Check sheet for the modelled part. Datum: model origin and axes. Units: mm. A direction names the side the tool comes from. Give positions to 0.01 mm unless a question says otherwise; leave off trailing zeros. Loops run counter-clockwise (first coordinate to the right, second up) from the corner with the lowest first, then second, coordinate; pieces in that order, holes last. Notation, with made-up numbers: (2.5, -23) - (35.5, -23) arc R22 ccw to (35.5, -4) - close; hole circle Ø5 at (46, 8.25). An arc over 180 degrees is marked (long way). Use CSV: the item, a comma, the result in double quotes.
from build123d import *

# Parameters (mm, degrees)
ESBO_O1_W                  = 90.2
ESBO_O1_H                  = 95.9
RESSALTO_EXTRUS_O1_DEPTH   = 3.5
ESBO_O2_R                  = 1.25
CORTE_EXTRUS_O1_DEPTH      = 5
CORTE_EXTRUS_O3_DEPTH      = 5
ESBO_O4_R                  = 1.25
CORTE_EXTRUS_O2_DEPTH      = 10
CHANFRO4_SIZE              = 1.75
CHANFRO5_SIZE              = 1.75
CHANFRO6_SIZE              = 2.25
CHANFRO7_SIZE              = 2.25
CORTE_EXTRUS_O4_DEPTH      = 0.2
CORTE_EXTRUS_O5_DEPTH      = 0.2
CORTE_EXTRUS_O7_DEPTH      = 66.920122118
CORTE_EXTRUS_O7_DEPTH_BACK = 5
ESBO_O7_W                  = 1.6
ESBO_O7_H                  = 6.5
ESBO_O8_W                  = 1.6
ESBO_O8_H                  = 6.5
CORTE_EXTRUS_O8_DEPTH      = 5


with BuildPart() as part:
    # Esboço1 → Ressalto-extrusão1 (new body)
    with BuildSketch(Plane.XY):
        Rectangle(ESBO_O1_W, ESBO_O1_H)
    extrude(amount=RESSALTO_EXTRUS_O1_DEPTH)

    # Esboço2 → Corte-extrusão1 (cut)
    with BuildSketch(Plane.XY):
        with Locations((-36.2, 42.85)):
            Circle(ESBO_O2_R)
        with Locations((37.5, 42.85)):
            Circle(ESBO_O2_R)
        with Locations((40, -42.85)):
            Circle(ESBO_O2_R)
        with Locations((-40, -42.85)):
            Circle(ESBO_O2_R)
    extrude(amount=CORTE_EXTRUS_O1_DEPTH, mode=Mode.SUBTRACT)

    # Esboço3 → Corte-extrusão3 (cut)
    with BuildSketch(Plane.XY):
        Polygon((-26.25, 41.25), (26.25, 41.25), (41.25, 26.25), (41.25, -26.25), (26.25, -41.25), (-26.25, -41.25), (-41.25, -26.25), (-41.25, 26.25), align=None)
    extrude(amount=CORTE_EXTRUS_O3_DEPTH, mode=Mode.SUBTRACT)

    # Esboço4 → Corte-extrusão2 (cut)
    with BuildSketch(Plane.XY):
        with Locations((-36.25, 36.25)):
            Circle(ESBO_O4_R)
        with Locations((36.25, 36.25)):
            Circle(ESBO_O4_R)
        with Locations((-36.25, -36.25)):
            Circle(ESBO_O4_R)
        with Locations((36.25, -36.25)):
            Circle(ESBO_O4_R)
    extrude(amount=CORTE_EXTRUS_O2_DEPTH, mode=Mode.SUBTRACT)

    # Chanfro4
    chanfro4_edges = [part.edges().sort_by_distance(p)[0] for p in [
        (-41.25, -42.85, 3.5),
    ]]
    chamfer(chanfro4_edges, length=CHANFRO4_SIZE)

    # Chanfro5
    chanfro5_edges = [part.edges().sort_by_distance(p)[0] for p in [
        (38.75, -42.85, 3.5),
    ]]
    chamfer(chanfro5_edges, length=CHANFRO5_SIZE)

    # Chanfro6
    chanfro6_edges = [part.edges().sort_by_distance(p)[0] for p in [
        (-37.45, 42.85, 3.5),
    ]]
    chamfer(chanfro6_edges, length=CHANFRO6_SIZE)

    # Chanfro7
    chanfro7_edges = [part.edges().sort_by_distance(p)[0] for p in [
        (36.25, 42.85, 3.5),
    ]]
    chamfer(chanfro7_edges, length=CHANFRO7_SIZE)

    # Esboço5 → Corte-extrusão4 (cut)
    with BuildSketch(Plane.XY.offset(3.5)):
        Polygon((-34.011664728, -41.359633286), (-33.364529311, -41.359633286), (-33.364529311, -44.859633286), (-33.678631875, -44.859633286), (-33.678631875, -41.718607645), (-34.217093414, -41.718607645), align=None)
    extrude(amount=-CORTE_EXTRUS_O4_DEPTH, mode=Mode.SUBTRACT)

    # Esboço6 → Corte-extrusão5 (cut)
    with BuildSketch(Plane(origin=(0, 0, 0), x_dir=(-1, 0, 0), z_dir=(0, 0, -1))):
        Polygon((33.93825461, -40.504659527), (34.585390027, -40.504659527), (34.585390027, -44.004659527), (34.271287463, -44.004659527), (34.271287463, -40.863633886), (33.732825924, -40.863633886), align=None)
    extrude(amount=-CORTE_EXTRUS_O5_DEPTH, mode=Mode.SUBTRACT)

    # Esboço7 → Corte-extrusão7 (cut, two sides: drawn at the far end of the back side and taken through both)
    with BuildSketch(Plane(origin=(0, 0, 0), x_dir=(-1, 0, 0), z_dir=(0, 0, -1)).offset(-CORTE_EXTRUS_O7_DEPTH_BACK)):
        with Locations((-44.3, -44.7)):
            Rectangle(ESBO_O7_W, ESBO_O7_H)
    extrude(amount=CORTE_EXTRUS_O7_DEPTH + CORTE_EXTRUS_O7_DEPTH_BACK, mode=Mode.SUBTRACT)

    # Esboço8 → Corte-extrusão8 (cut)
    with BuildSketch(Plane.XY.offset(3.5)):
        with Locations((-44.3, 44.7)):
            Rectangle(ESBO_O8_W, ESBO_O8_H)
    extrude(amount=-CORTE_EXTRUS_O8_DEPTH, mode=Mode.SUBTRACT)


solid = part.part
1. Release check for a two-part mould opening along Y. For faces 1 (the face through (0, 47.95, 2)), 2 (the face through (0, -41.25, 2)), 3 (the face through (0, -42, 0)) record: released by +Y, released by -Y, zero draft, split by the parting line, or undercut.
Completed:
face 1,"released by +Y"
face 2,"undercut"
face 3,"zero draft"
2. Sectioned sample at B-B, the plane y = -13.5. Record the boundary of the cut face in (x, z).
Completed:
outline,"(-45.1, 0) - (-41.25, 0) - (-41.25, 3.5) - (-45.1, 3.5) - close; (41.25, 0) - (45.1, 0) - (45.1, 3.5) - (41.25, 3.5) - close"
3. Scan lines: line 1 along Y through (x, z) = (-13.5, 3.3); line 2 along Y through (x, z) = (-36.25, 1.1); line 3 along X through (y, z) = (-42.85, 1.15). Record each from-to range of solid material in increasing order.
Completed:
line 1,"y = -47.95 to -41.25, 41.25 to 47.95"
line 2,"y = -47.95 to -37.5, -35 to -31.25, 31.25 to 35, 37.5 to 41.6, 44.1 to 47.95"
line 3,"x = -45.1 to -41.25, -38.75 to 38.75, 41.25 to 43.5"
4. Go/stop test with a flat-tipped pin: pin 1 Ø3 at (x, y) = (-40, -42.85) entering from +Z. Record where the tip stops, or that it passes through.
Completed:
pin 1,"stops at z = 2"
5. Sectioned sample at A-A, the plane x = -31.5. Record the boundary of the cut face in (y, z), and give its area (4 significant figures).
Completed:
outline,"(-47.95, 0) - (-36, 0) - (-36, 3.5) - (-47.95, 3.5) - close; (36, 0) - (47.95, 0) - (47.95, 3.5) - (36, 3.5) - close"
area,"83.65 mm²"
6. Set-up check for faces 4 (the face through (43.5, -45, 2)), 5 (the face through (-33.9, 33.6, 1.7)), 6 (the face through (-43.5, 45, 2)): record each of +Z, -Z, +X, -X, +Y, -Y from which the full face is reachable in a straight line by a thin tool's end or side.
Completed:
face 4,"+Z, -Z, +X, -Y"
face 5,"+Z, -Z"
face 6,"+Z, -Z, -X, +Y"
7. Sectioned sample at C-C, the plane y = -42.85. Record the boundary of the cut face in (x, z).
Completed:
outline,"(-45.1, 0) - (-41.25, 0) - (-41.25, 1.75) - (-43, 3.5) - (-45.1, 3.5) - close; (-38.75, 0) - (-34.59, 0) - (-34.59, 0.2) - (-34.27, 0.2) - (-34.27, 0) - (38.75, 0) - (38.75, 1.75) - (37, 3.5) - (-33.36, 3.5) - (-33.36, 3.3) - (-33.68, 3.3) - (-33.68, 3.5) - (-37, 3.5) - (-38.75, 1.75) - close; (41.25, 0) - (43.5, 0) - (43.5, 3.5) - (43, 3.5) - (41.25, 1.75) - close"
